```python
from build123d import *

# Parameters (mm, degrees)
BOSS_EXTRUDE2_DEPTH = 3
SKETCH4_R           = 2
SKETCH4_R_2         = 4
CUT_EXTRUDE3_DEPTH  = 7


with BuildPart() as part:
    # Sketch2 → Boss-Extrude2 (new body)
    with BuildSketch(Plane(origin=(0, 0, 0), x_dir=(1, 0, 0), z_dir=(0, 1, 0))):
        with BuildLine():
            Line((17.180375272, -22.928844638), (17.180375272, 33.071155362))
            ThreePointArc((17.180375272, 33.071155362), (14.401084996, 36.880337397), (9.925441387, 35.396108137))
            Line((9.925441387, 35.396108137), (-30.074558613, -20.603891863))
            ThreePointArc((-30.074558613, -20.603891863), (-30.376295299, -24.759170961), (-26.819624728, -26.928844638))
            Line((-26.819624728, -26.928844638), (13.180375272, -26.928844638))
            ThreePointArc((13.180375272, -26.928844638), (16.008802397, -25.757271762), (17.180375272, -22.928844638))
        make_face()
    extrude(amount=BOSS_EXTRUDE2_DEPTH)

    # Sketch4 → Cut-Extrude3 (cut)
    with BuildSketch(Plane(origin=(0, 0, 0), x_dir=(1, 0, 0), z_dir=(0, 1, 0))):
        with Locations(Location((13.180375272, -22.928844638, 0), (0, 0, 270))):
            Circle(SKETCH4_R)
        with Locations(Location((13.180375272, -14.928844638, 0), (0, 0, 270))):
            Circle(SKETCH4_R)
        with Locations(Location((13.180375272, -6.928844638, 0), (0, 0, 270))):
            Circle(SKETCH4_R)
        with Locations(Location((13.180375272, 1.071155362, 0), (0, 0, 270))):
            Circle(SKETCH4_R)
        with Locations(Location((13.180375272, 9.071155362, 0), (0, 0, 270))):
            Circle(SKETCH4_R)
        with Locations(Location((13.180375272, 17.071155362, 0), (0, 0, 270))):
            Circle(SKETCH4_R)
        with Locations(Location((13.180375272, 25.071155362, 0), (0, 0, 270))):
            Circle(SKETCH4_R)
        with Locations(Location((13.180375272, 33.071155362, 0), (0, 0, 270))):
            Circle(SKETCH4_R)
        with Locations(Location((5.180375272, -22.928844638, 0), (0, 0, 270))):
            Circle(SKETCH4_R)
        with Locations(Location((-2.819624728, -22.928844638, 0), (0, 0, 270))):
            Circle(SKETCH4_R)
        with Locations(Location((-10.819624728, -22.928844638, 0), (0, 0, 270))):
            Circle(SKETCH4_R)
        with Locations(Location((-18.819624728, -22.928844638, 0), (0, 0, 270))):
            Circle(SKETCH4_R)
        with Locations(Location((-26.819624728, -22.928844638, 0), (0, 0, 270))):
            Circle(SKETCH4_R)
        with Locations(Location((-18.819624728, -14.928844638, 0), (0, 0, 270))):
            Circle(SKETCH4_R)
        with Locations(Location((-10.819624728, -14.928844638, 0), (0, 0, 270))):
            Circle(SKETCH4_R)
        with Locations(Location((-2.819624728, -14.928844638, 0), (0, 0, 270))):
            Circle(SKETCH4_R)
        with Locations(Location((5.180375272, -14.928844638, 0), (0, 0, 270))):
            Circle(SKETCH4_R)
        with Locations(Location((5.180375272, -6.928844638, 0), (0, 0, 270))):
            Circle(SKETCH4_R)
        with Locations(Location((5.180375272, 1.071155362, 0), (0, 0, 270))):
            Circle(SKETCH4_R)
        with Locations(Location((5.180375272, 9.071155362, 0), (0, 0, 270))):
            Circle(SKETCH4_R)
        with Locations(Location((5.180375272, 17.071155362, 0), (0, 0, 270))):
            Circle(SKETCH4_R)
        with Locations(Location((-2.819624728, 1.071155362, 0), (0, 0, 270))):
            Circle(SKETCH4_R)
        with Locations(Location((-2.819624728, -6.928844638, 0), (0, 0, 270))):
            Circle(SKETCH4_R_2)
    extrude(amount=CUT_EXTRUDE3_DEPTH, mode=Mode.SUBTRACT)


solid = part.part
```
Geometry check sheet. Reference: the model listing, model coordinates, mm. Give positions to 0.01 mm unless a question says otherwise; leave off trailing zeros. Loops run counter-clockwise (first coordinate to the right, second up) from the corner with the lowest first, then second, coordinate; pieces in that order, holes last. Notation, with made-up numbers: (-19, 12) - (5, 12) arc R24 ccw to (5, 38) - close; hole circle Ø5 at (-21.5, 80). An arc over 180 degrees is marked (long way). Use CSV: the item, a comma, the result in double quotes. Start each with the question number.
Q1. Go/stop test with flat-tipped pins: pin 1 Ø2.5 at (x, z) = (5.18, -1.07) entering from +Y; pin 2 Ø1 at (y, z) = (0.5, -21.5) entering from -X; pin 3 Ø1 at (x, y) = (-7, 2) entering from -Z. Record where each tip stops, or that it passes through.
Q2. Section check A-A, the plane z = -8. Record the cut outline in (x, y), and give its area (3 significant figures).
Q3. Section check B-B, the plane x = -5.5. Record the cut outline in (y, z), and give its area (3 significant figures).
Q4. Scan lines: probe 1 along Z at (x, y) = (-3, 1.2); probe 2 along Z at (x, y) = (-12, 1.15); probe 3 along Z at (x, y) = (-10, 2.2). Record each from-to range of solid material in increasing order. Write a range as from..to.
Q5. Release check for a two-part mould opening along X. For faces 1 (the face through (15.978, 1.479, 25.788)), 2 (the face through (14.468, 1.479, -36.858)), 3 (the face through (-10.219, 1.479, 24.836)), 4 (the face through (-7, 1, 26.929)) record: +X half, -X half, draft (parallel to the pull), parting line (faces both ways), or undercut.
Q6. Section check D-D, the plane x = -12. Record the cut outline in (y, z), and give its area (3 significant figures).
Q7. Section check C-C, the plane z = 15. Record the cut outline in (x, y), and give its area (3 significant figures).
Findings below:
1,pin 1,"passes through"
1,pin 2,"stops at x = -0.36"
1,pin 3,"stops at z = -12.4"
2,outline,"(-9.64, 0) - (3.49, 0) - (3.49, 3) - (-9.64, 3) - close; (6.87, 0) - (11.49, 0) - (11.49, 3) - (6.87, 3) - close; (14.87, 0) - (17.18, 0) - (17.18, 3) - (14.87, 3) - close"
2,area,"60.2 mm^2"
3,outline,"(0, -13.8) - (3, -13.8) - (3, 3.96) - (0, 3.96) - close; (0, 9.9) - (3, 9.9) - (3, 26.93) - (0, 26.93) - close"
3,area,"104 mm^2"
4,probe 1,"z = -17.3..-3.06, 0.92..2.93, 10.92..12.94, 16.92..20.94, 24.92..26.93"
4,probe 2,"z = -4.7..13.31, 16.54..21.31, 24.54..26.93"
4,probe 3,"z = -7.5..13.1, 16.75..21.1, 24.75..26.93"
5,face 1,"+X half"
5,face 2,"parting line"
5,face 3,"undercut"
5,face 4,"draft"
6,outline,"(0, -4.7) - (3, -4.7) - (3, 13.31) - (0, 13.31) - close; (0, 16.54) - (3, 16.54) - (3, 21.31) - (0, 21.31) - close; (0, 24.54) - (3, 24.54) - (3, 26.93) - (0, 26.93) - close"
6,area,"75.5 mm^2"
7,outline,"(-26.07, 0) - (-20.82, 0) - (-20.82, 3) - (-26.07, 3) - close; (-16.82, 0) - (-12.82, 0) - (-12.82, 3) - (-16.82, 3) - close; (-8.82, 0) - (-4.82, 0) - (-4.82, 3) - (-8.82, 3) - close; (-0.82, 0) - (3.18, 0) - (3.18, 3) - (-0.82, 3) - close; (7.18, 0) - (11.18, 0) - (11.18, 3) - (7.18, 3) - close; (15.18, 0) - (17.18, 0) - (17.18, 3) - (15.18, 3) - close"
7,area,"69.8 mm^2"
